Part model, mm, in its own coordinate system. Face numbers are marked on the shaded views. Give positions to 0.01 mm unless a question says otherwise; leave off trailing zeros. Order: outer loops, then holes, each group sorted by start corner. A loop starts at its lowest first (then second) coordinate and runs counter-clockwise, first axis right, second up. Notation, with made-up numbers: M 11.25,13 L 31.25,13 A25 ccw 31.25,40 Z; hole C 44,-14 d1. An arc over 180 degrees is marked long. Return JSON: item names as keys, results as strings.
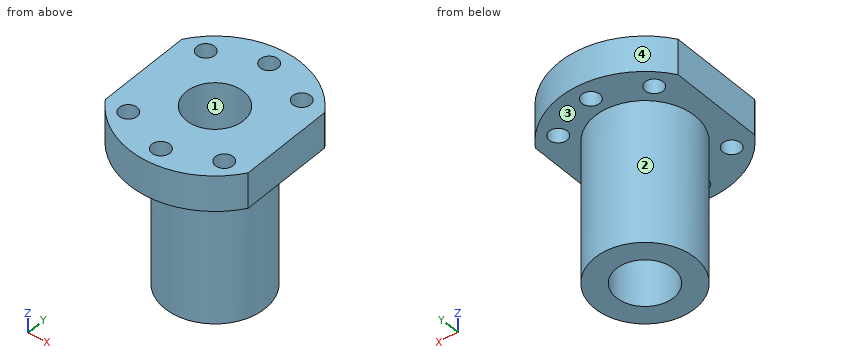
from build123d import *

# Parameters (mm, degrees)
SCHIZZO1_R                   = 8
SCHIZZO1_R_2                 = 2.5
ESTRUSIONE_ESTRUSIONE1_DEPTH = 50
SCHIZZO2_OUTSIDE_W           = 58.004
SCHIZZO2_OUTSIDE_H           = 66.004
SCHIZZO2_OUTSIDE_R           = 14
TAGLIO_ESTRUSIONE1_DEPTH     = 40


with BuildPart() as part:
    # Schizzo1 → Estrusione-Estrusione1 (new body)
    with BuildSketch(Plane.XY):
        with BuildLine():
            Line((20, -13.266499161), (20, 13.266499161))
            ThreePointArc((20, 13.266499161), (0, 24), (-20, 13.266499161))
            Line((-20, 13.266499161), (-20, -13.266499161))
            ThreePointArc((-20, -13.266499161), (0, -24), (20, -13.266499161))
        make_face()
        Circle(SCHIZZO1_R, mode=Mode.SUBTRACT)
        with Locations((-13.435028843, 13.435028843)):
            Circle(SCHIZZO1_R_2, mode=Mode.SUBTRACT)
        with Locations((13.435028843, 13.435028843)):
            Circle(SCHIZZO1_R_2, mode=Mode.SUBTRACT)
        with Locations((13.435028843, -13.435028843)):
            Circle(SCHIZZO1_R_2, mode=Mode.SUBTRACT)
        with Locations((-13.435028843, -13.435028843)):
            Circle(SCHIZZO1_R_2, mode=Mode.SUBTRACT)
        with Locations((0, 18.781867411)):
            Circle(SCHIZZO1_R_2, mode=Mode.SUBTRACT)
        with Locations((0, -18.781867411)):
            Circle(SCHIZZO1_R_2, mode=Mode.SUBTRACT)
    extrude(amount=-ESTRUSIONE_ESTRUSIONE1_DEPTH)

    # Schizzo2 outside → Taglio-Estrusione1 (cut)
    with BuildSketch(Plane(origin=(0, 0, -50), x_dir=(-1, 0, 0), z_dir=(0, 0, -1))):
        Rectangle(SCHIZZO2_OUTSIDE_W, SCHIZZO2_OUTSIDE_H)
        Circle(SCHIZZO2_OUTSIDE_R, mode=Mode.SUBTRACT)
    extrude(amount=-TAGLIO_ESTRUSIONE1_DEPTH, mode=Mode.SUBTRACT)


solid = part.part
Q1. Pin check, flat tips, straight feed: pin 1 (4.5 mm diameter, centred on x = 13.44, y = 13.44, fed in from -Z); pin 2 (12 mm diameter, centred on x = -1.5, y = -3, fed in from -Z); pin 3 (4 mm diameter, centred on x = 12.5, z = -17, fed in from +Y); pin 4 (5 mm diameter, centred on x = 7.5, z = -18, fed in from -Y). Stop position of each tip, or through.
Established:
{"pin 1": "passes through", "pin 2": "stops at z = -50", "pin 3": "stops at y = 9.26", "pin 4": "stops at y = -13.08"}
Q2. Band-saw the part on D-D (x = -4). Give the cut face in (y, z), then the cut area to 3 significant figures.
Established:
{"outline": "M -23.66,-10 L -13.42,-10 L -13.42,-50 L -6.93,-50 L -6.93,0 L -23.66,0 Z; M 6.93,-50 L 13.42,-50 L 13.42,-10 L 23.66,-10 L 23.66,0 L 6.93,0 Z", "area": "854 mm²"}
Q3. Band-saw the part on B-B (y = 0). Give the cut face in (x, z).
Established:
{"outline": "M -20,-10 L -14,-10 L -14,-50 L -8,-50 L -8,0 L -20,0 Z; M 8,-50 L 14,-50 L 14,-10 L 20,-10 L 20,0 L 8,0 Z"}
Q4. Band-saw the part on A-A (x = 0). Give the cut face in (y, z).
Established:
{"outline": "M -24,-10 L -21.28,-10 L -21.28,0 L -24,0 Z; M -16.28,-10 L -14,-10 L -14,-50 L -8,-50 L -8,0 L -16.28,0 Z; M 8,-50 L 14,-50 L 14,-10 L 16.28,-10 L 16.28,0 L 8,0 Z; M 21.28,-10 L 24,-10 L 24,0 L 21.28,0 Z"}
Q5. Band-saw the part on C-C (z = -4.5). Give the cut face in (x, y), then the cut area to 3 significant figures.
Established:
{"outline": "M -20,-13.27 A24 ccw 20,-13.27 L 20,13.27 A24 ccw -20,13.27 Z; hole C -13.44,-13.44 d5; hole C -13.44,13.44 d5; hole C 0,0 d16; hole C 0,-18.78 d5; hole C 0,18.78 d5; hole C 13.44,-13.44 d5; hole C 13.44,13.44 d5", "area": "1,350 mm²"}
Q6. Two-plate mould, pull along Y, no slides. Class the marked faces 1, 2, 3 and 4: +Y half, -Y half, draft (parallel to the pull), parting line (faces both ways), or undercut.
Established:
{"face 1": "undercut", "face 2": "parting line", "face 3": "draft", "face 4": "+Y half"}
Q7. Probe line 1 along Y through (x, z) = (0, -22); line 2 along Z through (x, y) = (12, -20); line 3 along Y through (x, z) = (-3.5, -15). List the from-to ranges inside material, lowest first.
Established:
{"line 1": "y = -14 to -8, 8 to 14", "line 2": "z = -10 to 0", "line 3": "y = -13.56 to -7.19, 7.19 to 13.56"}
